For this review, take the finished solid that the model builds, in its own axes (mm). Face numbers are marked on the shaded views. A direction names the side the tool comes from. Round coordinates to 2 decimals unless told otherwise and drop trailing zeros. Write each loop counter-clockwise with the first axis right and the second up, starting at its lowest first coordinate (ties: lowest second). Pieces come first, ordered by that corner, then holes. Notation, with made-up numbers: M 28,33.5 L 63,33.5 A17 ccw 63,49.5 Z; hole C -7.75,28.5 d2. An arc over 180 degrees is marked long. Answer in a Markdown table with one row per item.
```python
from build123d import *

# Parameters (mm, degrees)
SKETCH1_W           = 20
SKETCH1_H           = 20
BOSS_EXTRUDE1_DEPTH = 3
SKETCH2_W           = 3.5
SKETCH2_H           = 20
BOSS_EXTRUDE2_DEPTH = 12
SKETCH3_R           = 3
CUT_EXTRUDE1_DEPTH  = 12
FILLET1_R           = 2
SKETCH4_R           = 1.5
CUT_EXTRUDE2_DEPTH  = 12


with BuildPart() as part:
    # Sketch1 → Boss-Extrude1 (new body)
    with BuildSketch(Plane(origin=(0, 0, 0), x_dir=(1, 0, 0), z_dir=(0, 1, 0))):
        Rectangle(SKETCH1_W, SKETCH1_H)
    extrude(amount=BOSS_EXTRUDE1_DEPTH)

    # Sketch2 → Boss-Extrude2 (add)
    with BuildSketch(Plane(origin=(0, 3, 0), x_dir=(1, 0, 0), z_dir=(0, 1, 0))):
        with Locations((-8.25, 0)):
            Rectangle(SKETCH2_W, SKETCH2_H)
    extrude(amount=BOSS_EXTRUDE2_DEPTH)

    # Sketch3 → Cut-Extrude1 (cut)
    with BuildSketch(Plane.ZY.offset(10)):
        with Locations((0, 10)):
            Circle(SKETCH3_R)
    extrude(amount=-CUT_EXTRUDE1_DEPTH, mode=Mode.SUBTRACT)

    # Fillet1
    fillet1_edges = [part.edges().sort_by_distance(p)[0] for p in [
        (10, 1.5, -10),
        (10, 1.5, 10),
    ]]
    fillet(fillet1_edges, radius=FILLET1_R)

    # Sketch4 → Cut-Extrude2 (cut)
    with BuildSketch(Plane(origin=(0, 3, 0), x_dir=(1, 0, 0), z_dir=(0, 1, 0))):
        with Locations(Location((2, 6.060166803, 0), (0, 0, 270))):
            Circle(SKETCH4_R)
        with Locations(Location((2, -6.359845381, 0), (0, 0, 270))):
            Circle(SKETCH4_R)
    extrude(amount=-CUT_EXTRUDE2_DEPTH, mode=Mode.SUBTRACT)


solid = part.part
```
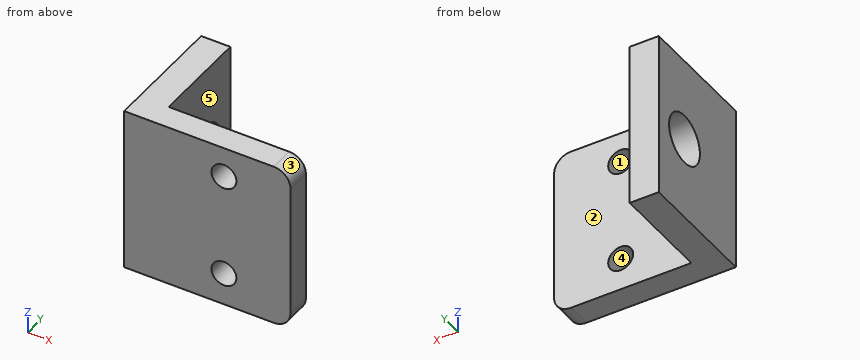
Q1. Mouldability with a two-part tool opening along Z and no side actions: class the marked faces 1, 2 and 3 as +Z half, -Z half, draft (parallel to the pull), parting line (faces both ways), or undercut.
Found:
| item | result |
|---|---|
| face 1 | undercut |
| face 2 | draft |
| face 3 | +Z half |
Q2. Take a section at D-D (x = -7.25). State the section outline as (y, z) points, then the cut area to 3 significant figures.
Found:
| item | result |
|---|---|
| outline | M 0,-10 L 15,-10 L 15,10 L 0,10 Z; hole C 10,0 d6 |
| area | 272 mm² |
Q3. Take a section at B-B (y = 10). State the section outline as (x, z) points, then the cut area to 3 significant figures.
Found:
| item | result |
|---|---|
| outline | M -10,-10 L -6.5,-10 L -6.5,-3 L -10,-3 Z; M -10,3 L -6.5,3 L -6.5,10 L -10,10 Z |
| area | 49.0 mm² |
Q4. Take a section at C-C (z = 0). State the section outline as (x, y) points, then the cut area to 3 significant figures.
Found:
| item | result |
|---|---|
| outline | M -10,0 L 10,0 L 10,3 L -6.5,3 L -6.5,7 L -10,7 Z; M -10,13 L -6.5,13 L -6.5,15 L -10,15 Z |
| area | 81.0 mm² |
Q5. Take a section at A-A (x = 2). State the section outline as (y, z) points, then the cut area to 3 significant figures.
Found:
| item | result |
|---|---|
| outline | M 0,-10 L 3,-10 L 3,-7.56 L 0,-7.56 Z; M 0,-4.56 L 3,-4.56 L 3,4.86 L 0,4.86 Z; M 0,7.86 L 3,7.86 L 3,10 L 0,10 Z |
| area | 42.0 mm² |
Q6. Insertion check: P1, Ø12, axis at x = 7, z = 0, coming from the +Y side. The pin has a flat end and moves straight along its axis. Give the tip position at first contact, or say it passes through.
Found:
| item | result |
|---|---|
| P1 | y = 3 |
Q7. Machinability: for the marked faces 4 and 5, which of the approach directions +Z, -Z, +X, -X, +Y, -Y give a long, thin tool a straight path to every point of the face, cutting with its end or side? Answer none if there is none.
Found:
| item | result |
|---|---|
| face 4 | +Y, -Y |
| face 5 | +Z, -Z, +X, +Y |
Q8. For probe 1 along X at (y, z) = (6.25, -2); probe 2 along Y at (x, z) = (-6, -7); probe 3 along X at (y, z) = (2.75, 6.25), list the stretches that pass through material, from the lowest coordinate up.
Found:
| item | result |
|---|---|
| probe 1 | -10 to -6.5 |
| probe 2 | 0 to 3 |
| probe 3 | -10 to 0.5, 3.5 to 10 |
